Build history of the part. All positions in model axes, mm. A direction names the side the tool comes from. Round coordinates to 2 decimals unless told otherwise and drop trailing zeros. Loops run counter-clockwise (first coordinate to the right, second up) from the corner with the lowest first, then second, coordinate; pieces in that order, holes last. Notation, with made-up numbers: (36.5, 39) -> (66.5, 39) arc R13 ccw to (66.5, 49) -> close; hole circle Ø5 at (58.25, 49.5). An arc over 180 degrees is marked (long way). Put each result on its own line as item: value. Start each with the question number.
Item 1: Drill centre lines: probe 1 along X at (y, z) = (-2.25, -4.5); probe 2 along Y at (x, z) = (-12, -10); probe 3 along X at (y, z) = (-0.5, -7). Where is each one in solid material? Low to high. Write a range as [from, to].
Item 2: Cut at A-A, the plane z = 0. List the corners of the cut face in (x, y).
Item 3: Cut at D-D, the plane y = -12.5. List the corners of the cut face in (x, z).
Item 4: Pull direction X, two halves, no side cores. Call faces 1 (the flat face through (38, -13.5, -3)), 2 (the cylindrical face through (-27.07, -12.9, -5.09)), 3 (the cylindrical face through (-26.05, -14, 5.16)): +X half, -X half, draft (parallel to the pull), parting line (faces both ways), or undercut.
Item 5: Cut at B-B, the plane y = -3.5. List the corners of the cut face in (x, z).
Item 6: Flat gauge pins, fed straight in: pin 1 Ø6 at (x, z) = (14, -3) entering from -Y; pin 2 Ø3.5 at (x, y) = (-35.5, -12.5) entering from -Z; pin 3 Ø1.2 at (x, z) = (25.5, -0.5) entering from -Y; pin 4 Ø6 at (y, z) = (-4, -23.5) entering from -X. Where does each tip first touch, or does it go through?
Item 7: Tool access for faces 4 (the flat face through (0, 1.5, -15)), 5 (the cylindrical face through (15, 0.7, -17.5)), 6 (the cylindrical face through (20.86, 0.74, -8.4)), 7 (the flat face through (26.5, -7, 0)), 8 (the flat face through (25, -7, 0)): list every direction of +Z, -Z, +X, -X, +Y, -Y with a clear straight run to the whole face (end or side of a thin tool).
Item 8: Cut at C-C, the plane x = -35. List the corners of the cut face in (y, z), plus the area to 4 significant figures.
```python
from build123d import *

# Parameters (mm, degrees)
ODGI_CIE_BAZOWE1_DEPTH      = 7.5
SZCZELINA_START             = -15
SZCZELINA_POD_RUB_M51_DEPTH = 1.5
SZKIC8_W                    = 40
SZKIC8_H                    = 30
WYPUST1_DEPTH               = 1.5
SZCZELINA_POD_RUB_M31_DEPTH = 1.5
SZKIC13_W                   = 4.75
SZKIC13_H                   = 5.5
WYTNIJ_WYCI_GNI_CIE1_DEPTH  = 7
ZAOKR_GLENIE1_R             = 3


# Read off the part's stored shape, not the designer's step: Szczelina pod śrubę M51, Szczelina pod śrubę M31
# Sheet-metal steps are written as plain solids
with BuildPart() as part:
    # Szkic1 → Odgięcie bazowe1 (new, symmetric)
    with BuildSketch(Plane.XY):
        with BuildLine():
            Line((-48, -15), (-28.5, -15))
            ThreePointArc((-28.5, -15), (-26.025126266, -13.974873734), (-25, -11.5))
            Line((-25, -11.5), (-25, -2))
            ThreePointArc((-25, -2), (-24.414213562, -0.585786438), (-23, 0))
            Line((-23, 0), (23, 0))
            ThreePointArc((23, 0), (24.414213562, -0.585786438), (25, -2))
            Line((25, -2), (25, -11.5))
            ThreePointArc((25, -11.5), (26.025126266, -13.974873734), (28.5, -15))
            Line((28.5, -15), (48, -15))
            Line((48, -15), (48, -13.5))
            Line((48, -13.5), (28.5, -13.5))
            ThreePointArc((28.5, -13.5), (27.085786438, -12.914213562), (26.5, -11.5))
            Line((26.5, -11.5), (26.5, -2))
            ThreePointArc((26.5, -2), (25.474873734, 0.474873734), (23, 1.5))
            Line((23, 1.5), (-23, 1.5))
            ThreePointArc((-23, 1.5), (-25.474873734, 0.474873734), (-26.5, -2))
            Line((-26.5, -2), (-26.5, -11.5))
            ThreePointArc((-26.5, -11.5), (-27.085786438, -12.914213562), (-28.5, -13.5))
            Line((-28.5, -13.5), (-48, -13.5))
            Line((-48, -13.5), (-48, -15))
        make_face()
    extrude(amount=ODGI_CIE_BAZOWE1_DEPTH, both=True)

    # Szczelina pod śrubę M51 outline → Szczelina pod śrubę M51 (cut)
    with BuildSketch(Plane(origin=(0, 0, 0), x_dir=(1, 0, 0), z_dir=(0, 1, 0)).offset(SZCZELINA_START)):
        with BuildLine():
            Line((29.75, -2.75), (40.25, -2.75))
            ThreePointArc((40.25, -2.75), (43, 0), (40.25, 2.75))
            Line((40.25, 2.75), (29.75, 2.75))
            ThreePointArc((29.75, 2.75), (27, 0), (29.75, -2.75))
        make_face()
        with BuildLine():
            ThreePointArc((-29.75, -2.75), (-27, 0), (-29.75, 2.75))
            Line((-29.75, 2.75), (-40.25, 2.75))
            ThreePointArc((-40.25, 2.75), (-43, 0), (-40.25, -2.75))
            Line((-40.25, -2.75), (-29.75, -2.75))
        make_face()
    extrude(amount=SZCZELINA_POD_RUB_M51_DEPTH, mode=Mode.SUBTRACT)

    # Szkic8 → Wypust1 (add)
    with BuildSketch(Plane(origin=(0, 1.5, 0), x_dir=(1, 0, 0), z_dir=(0, 1, 0))):
        with Locations((0, 22.5)):
            Rectangle(SZKIC8_W, SZKIC8_H)
    extrude(amount=-WYPUST1_DEPTH)

    # Szczelina pod śrubę M31 outline → Szczelina pod śrubę M31 (cut)
    with BuildSketch(Plane(origin=(0, 0, 0), x_dir=(1, 0, 0), z_dir=(0, 1, 0))):
        with BuildLine():
            Line((-13.3, 15.8), (13.3, 15.8))
            ThreePointArc((13.3, 15.8), (15, 17.5), (13.3, 19.2))
            Line((13.3, 19.2), (-13.3, 19.2))
            ThreePointArc((-13.3, 19.2), (-15, 17.5), (-13.3, 15.8))
        make_face()
    extrude(amount=SZCZELINA_POD_RUB_M31_DEPTH, mode=Mode.SUBTRACT)

    # Szkic13 → Wytnij-wyciągnięcie1 (cut)
    with BuildSketch(Plane.XZ.offset(15)):
        with Locations((-27.375, 0)):
            Rectangle(SZKIC13_W, SZKIC13_H)
        with Locations((27.375, 0)):
            Rectangle(SZKIC13_W, SZKIC13_H)
    extrude(amount=-WYTNIJ_WYCI_GNI_CIE1_DEPTH, mode=Mode.SUBTRACT)

    # Zaokrąglenie1
    zaokr_glenie1_edges = [part.edges().sort_by_distance(p)[0] for p in [
        (48, -14.25, 7.5),
        (48, -14.25, -7.5),
        (20, 0.75, -37.5),
        (-20, 0.75, -37.5),
        (-48, -14.25, -7.5),
        (-48, -14.25, 7.5),
        (20, 0.75, -7.5),
        (-20, 0.75, -7.5),
    ]]
    fillet(zaokr_glenie1_edges, radius=ZAOKR_GLENIE1_R)


solid = part.part
```
Reply:
1. probe 1: x = [-26.5, -25], [25, 26.5]
1. probe 2: y = [0, 1.5]
1. probe 3: x = [-26.16, -24.32], [24.32, 26.16]
2. outline: (-48, -15) -> (-43, -15) -> (-43, -13.5) -> (-48, -13.5) -> close; (-26.5, -8) -> (-25, -8) -> (-25, -2) arc R2 cw to (-23, 0) -> (23, 0) arc R2 cw to (25, -2) -> (25, -8) -> (26.5, -8) -> (26.5, -2) arc R3.5 ccw to (23, 1.5) -> (-23, 1.5) arc R3.5 ccw to (-26.5, -2) -> close; (43, -15) -> (48, -15) -> (48, -13.5) -> (43, -13.5) -> close
3. outline: (-26.77, -7.5) -> (-25.15, -7.5) -> (-25.15, -2.75) -> (-26.77, -2.75) -> close; (-26.77, 2.75) -> (-25.15, 2.75) -> (-25.15, 7.5) -> (-26.77, 7.5) -> close; (25.15, -7.5) -> (26.77, -7.5) -> (26.77, -2.75) -> (25.15, -2.75) -> close; (25.15, 2.75) -> (26.77, 2.75) -> (26.77, 7.5) -> (25.15, 7.5) -> close
4. face 1: draft
4. face 2: -X half
4. face 3: undercut
5. outline: (-26.5, -7.5) -> (-25, -7.5) -> (-25, 7.5) -> (-26.5, 7.5) -> close; (25, -7.5) -> (26.5, -7.5) -> (26.5, 7.5) -> (25, 7.5) -> close
6. pin 1: stops at y = 0
6. pin 2: stops at z = -7.5
6. pin 3: stops at y = -8
6. pin 4: passes through
7. face 4: +Z, -Z, +X, -X, +Y
7. face 5: +Y, -Y
7. face 6: -Z, +X, +Y, -Y
7. face 7: +Z, -Z, +X, +Y
7. face 8: +Z, -Z, -Y
8. outline: (-15, -7.5) -> (-13.5, -7.5) -> (-13.5, -2.75) -> (-15, -2.75) -> close; (-15, 2.75) -> (-13.5, 2.75) -> (-13.5, 7.5) -> (-15, 7.5) -> close
8. area: 14.25 mm^2
